from build123d import *

# Parameters (mm, degrees)
BOSS_EXTRUDE1_START                = -15.24
SKETCH2_R                          = 60.96
SKETCH2_R_2                        = 53.34
BOSS_EXTRUDE1_DEPTH                = 15.24
F_1_16_NPT_TAPPED_HOLE2_AT_2_COUNT = 2
F_1_16_NPT_TAPPED_HOLE2_AT_2_PITCH = 58.42
F_1_16_NPT_TAPPED_HOLE2_AT_3_COUNT = 2
F_1_16_NPT_TAPPED_HOLE2_AT_3_PITCH = 101.186408178
F_1_16_NPT_TAPPED_HOLE2_AT_4_COUNT = 2
F_1_16_NPT_TAPPED_HOLE2_AT_4_PITCH = 116.84
F_1_16_NPT_TAPPED_HOLE2_AT_5_COUNT = 2
F_1_16_NPT_TAPPED_HOLE2_AT_5_PITCH = 101.186408178
F_1_16_NPT_TAPPED_HOLE2_AT_6_COUNT = 2
F_1_16_NPT_TAPPED_HOLE2_AT_6_PITCH = 58.42
SKETCH8_R                          = 25.4
CUT_EXTRUDE1_DEPTH                 = 2.54


with BuildPart() as part:
    # Sketch1 → Revolve1 (revolve)
    with BuildSketch(Plane.XY, mode=Mode.PRIVATE) as revolve1_sk:
        with BuildLine():
            Line((0, 0), (60.96, 0))
            Line((60.96, 0), (60.96, -2.54))
            ThreePointArc((60.96, -2.54), (62.756051224, -1.796051224), (63.5, 0))
            Line((63.5, 0), (63.5, 127))
            Line((63.5, 127), (60.96, 127))
            Line((60.96, 127), (60.96, 2.54))
            Line((60.96, 2.54), (0, 2.54))
            Line((0, 2.54), (0, 0))
        make_face()
    revolve(revolve1_sk.sketch.rotate(Axis((0, 0, 0), (0, 1, 0)), 90), axis=Axis((0, 0, 0), (0, 1, 0)))

    # Sketch2 → Boss-Extrude1 (add)
    with BuildSketch(Plane(origin=(0, 127, 0), x_dir=(1, 0, 0), z_dir=(0, 1, 0)).offset(BOSS_EXTRUDE1_START)):
        with Locations(Location((0, 0, 0), (0, 0, 90))):
            Circle(SKETCH2_R)
        with Locations(Location((0, 0, 0), (0, 0, 270))):
            Circle(SKETCH2_R_2, mode=Mode.SUBTRACT)
    extrude(amount=BOSS_EXTRUDE1_DEPTH)

    # Sketch7 → 1/16 NPT Tapped Hole2 (revolve, cut)
    with BuildSketch(Plane(origin=(0, 127, -58.42), x_dir=(0, 0, 1), z_dir=(1, 0, 0))):
        Polygon((0, 0), (0, 13.530685027), (3.0734, 11.684), (3.0734, 6.858), (3.364810096, 6.858), (3.5701478, 0), align=None)
    f_1_16_npt_tapped_hole2 = revolve(axis=Axis((0, 133.35, -58.42), (0, -1, 0)), mode=Mode.SUBTRACT)

    # 1/16 NPT Tapped Hole2 at 2: 1/16 NPT Tapped Hole2 ×2
    with Locations(*[Vector(-0.8660254037844416, 0, 0.499999999999995) * (i * F_1_16_NPT_TAPPED_HOLE2_AT_2_PITCH) for i in range(1, F_1_16_NPT_TAPPED_HOLE2_AT_2_COUNT)]):
        add(f_1_16_npt_tapped_hole2, mode=Mode.SUBTRACT)

    # 1/16 NPT Tapped Hole2 at 3: 1/16 NPT Tapped Hole2 ×2
    with Locations(*[Vector(-0.5000000000000038, 0, 0.8660254037844365) * (i * F_1_16_NPT_TAPPED_HOLE2_AT_3_PITCH) for i in range(1, F_1_16_NPT_TAPPED_HOLE2_AT_3_COUNT)]):
        add(f_1_16_npt_tapped_hole2, mode=Mode.SUBTRACT)

    # 1/16 NPT Tapped Hole2 at 4: 1/16 NPT Tapped Hole2 ×2
    with Locations(*[(0, 0, i * F_1_16_NPT_TAPPED_HOLE2_AT_4_PITCH) for i in range(1, F_1_16_NPT_TAPPED_HOLE2_AT_4_COUNT)]):
        add(f_1_16_npt_tapped_hole2, mode=Mode.SUBTRACT)

    # 1/16 NPT Tapped Hole2 at 5: 1/16 NPT Tapped Hole2 ×2
    with Locations(*[Vector(0.49999999999999206, 0, 0.8660254037844433) * (i * F_1_16_NPT_TAPPED_HOLE2_AT_5_PITCH) for i in range(1, F_1_16_NPT_TAPPED_HOLE2_AT_5_COUNT)]):
        add(f_1_16_npt_tapped_hole2, mode=Mode.SUBTRACT)

    # 1/16 NPT Tapped Hole2 at 6: 1/16 NPT Tapped Hole2 ×2
    with Locations(*[Vector(0.8660254037844346, 0, 0.500000000000007) * (i * F_1_16_NPT_TAPPED_HOLE2_AT_6_PITCH) for i in range(1, F_1_16_NPT_TAPPED_HOLE2_AT_6_COUNT)]):
        add(f_1_16_npt_tapped_hole2, mode=Mode.SUBTRACT)

    # Sketch8 → Cut-Extrude1 (cut)
    with BuildSketch(Plane.XZ):
        with Locations(Location((0, 0, 0), (0, 0, 270))):
            Circle(SKETCH8_R)
    extrude(amount=-CUT_EXTRUDE1_DEPTH, mode=Mode.SUBTRACT)


solid = part.part
Here's how the part is built. I have some questions about the finished solid (model axes, mm). A direction names the side the tool comes from. Give positions to 0.01 mm unless a question says otherwise; leave off trailing zeros. Loops run counter-clockwise (first coordinate to the right, second up) from the corner with the lowest first, then second, coordinate; pieces in that order, holes last. Notation, with made-up numbers: (38, 79.5) -> (44, 79.5) arc R19 ccw to (44, 92.5) -> close; hole circle Ø11 at (84, 22.25). An arc over 180 degrees is marked (long way). One line per item, written item: value.
Q1. On a 3-axis mill with a long thin cutter (end or side, diameter ignored), from which of +Z, -Z, +X, -X, +Y, -Y can I reach the whole of each face in a straight line? I mean faces 1 (the face through (54, 111.76, 0)), 2 (the face through (26, 0, -1)), 3 (the face through (-15.456, 1.252, 20.157)), 4 (the face through (-53.185, 117.763, 30.862)). Say none if no direction works.
Answers follow:
face 1: none
face 2: -Y
face 3: +Y, -Y
face 4: +Y
Q2. We'd pull the mould along Z, two halves only. Please class faces 5 (the face through (61.99, 64.39, 13.77)), 6 (the face through (-51.12, 113.79, -29.28)): pulls with the +Z half, pulls with the -Z half, needs draft (parallel to the pull), parting line crosses it, or undercut.
Answers follow:
face 5: parting line crosses it
face 6: undercut
Q3. If I drill on line 1 along Y through (x, z) = (18, -51); line 2 along X through (y, z) = (48.5, 0); line 3 along Z through (x, y) = (1, 55), over which ranges is the centre line in solid material (lowest first)?
Answers follow:
line 1: 0 to 2.54, 111.76 to 127
line 2: -63.5 to -60.96, 60.96 to 63.5
line 3: -63.49 to -60.95, 60.95 to 63.49
Q4. Suppose I cut it at A-A on z = 0. Please give me the cut outline in (x, y), then the cut area to 3 significant figures.
Answers follow:
outline: (-63.5, 0) arc R2.54 ccw to (-60.96, -2.54) -> (-60.96, 0) -> (-25.4, 0) -> (-25.4, 2.54) -> (-60.96, 2.54) -> (-60.96, 111.76) -> (-53.34, 111.76) -> (-53.34, 127) -> (-63.5, 127) -> close; (25.4, 0) -> (60.96, 0) -> (60.96, -2.54) arc R2.54 ccw to (63.5, 0) -> (63.5, 127) -> (53.34, 127) -> (53.34, 111.76) -> (60.96, 111.76) -> (60.96, 2.54) -> (25.4, 2.54) -> close
area: 1,070 mm^2
Q5. I'm going to push flat-ended pins straight in: pin 1 Ø1.5 at (x, y) = (22, 107.5) entering from +Z; pin 2 Ø1 at (x, y) = (-33, 38) entering from -Z; pin 3 Ø5 at (x, y) = (-14, 37.5) entering from +Z. Where does each tip first touch, or does it pass through?
Answers follow:
pin 1: z = 59.84
pin 2: z = -54.55
pin 3: z = 62.45
Q6. Suppose I cut it at B-B on y = 109. Please give me the cut outline in (x, z), then the cut area to 3 significant figures.
Answers follow:
outline: circle Ø127 at (0, 0); hole circle Ø121.92 at (0, 0)
area: 993 mm^2
